Part model, mm, in its own coordinate system. Face numbers are marked on the shaded views. A direction names the side the tool comes from. Round coordinates to 2 decimals unless told otherwise and drop trailing zeros. Order: outer loops, then holes, each group sorted by start corner. A loop starts at its lowest first (then second) coordinate and runs counter-clockwise, first axis right, second up. Notation, with made-up numbers: (-24.5, 65.5) - (-8.5, 65.5) arc R35 cw to (-8.5, 100.5) - close; hole circle Ø3 at (-28.5, 24). An arc over 180 degrees is marked (long way). Return JSON: item names as keys, results as strings. Group by question number.
Item 1: Saw through at A-A on z = 0. List the corners of the cut face in (x, y).
Item 2: Saw through at B-B on x = 0. List the corners of the cut face in (y, z).
Item 3: Tool access for the marked faces 4 and 5: list every direction of +Z, -Z, +X, -X, +Y, -Y with a clear straight run to the whole face (end or side of a thin tool).
Item 4: Probe probe 1 along X at (y, z) = (2.3, -5.75); probe 2 along X at (y, z) = (1.8, -6). List the from-to ranges inside material, lowest first.
Item 5: Drop flat-ended pins along their axis: pin 1 (1.8 mm diameter, centred on x = 4.95, z = 4.95, fed in from +Y); pin 2 (4 mm diameter, centred on x = -4.95, z = -4.95, fed in from -Y); pin 3 (5 mm diameter, centred on x = 0, z = 0, fed in from -Y); pin 4 (1.5 mm diameter, centred on y = 0, z = 4, fed in from -X). Give the stop position or say it passes through.
Item 6: Saw through at C-C on z = -4.25. List the corners of the cut face in (x, y), and give its area (3 significant figures).
Item 7: Saw through at D-D on y = -1.1. List the corners of the cut face in (x, z).
Item 8: Two-plate mould, pull along X, no slides. Class the marked faces 1, 2 and 3: released by +X, released by -X, zero draft, split by the parting line, or undercut.
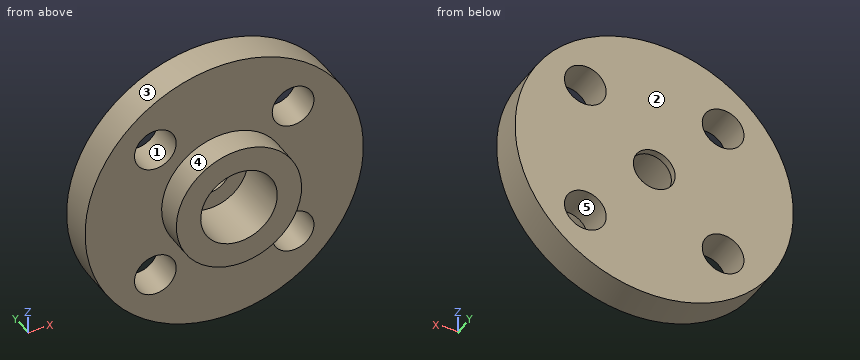
```python
from build123d import *

# Parameters (mm, degrees)
SKETCH_1_R          = 10
SKETCH_1_R_2        = 1.5
EXTRUDE_1_DEPTH     = 2.5
SKETCH_2_R          = 4.5
EXTRUDE_2_DEPTH     = 2
SKETCH_3_R          = 2.75
CUT_EXTRUDE_1_DEPTH = 4


with BuildPart() as part:
    # 草图1 → 凸台-拉伸1 (new body)
    with BuildSketch(Plane(origin=(0, 0, 0), x_dir=(1, 0, 0), z_dir=(0, 1, 0))):
        with Locations(Location((0, 0, 0), (0, 0, 270))):
            Circle(SKETCH_1_R)
        with Locations(Location((0, 0, 0), (0, 0, 270))):
            Circle(SKETCH_1_R_2, mode=Mode.SUBTRACT)
        with Locations(Location((-4.949747468, 4.949747468, 0), (0, 0, 270))):
            Circle(SKETCH_1_R_2, mode=Mode.SUBTRACT)
        with Locations(Location((4.949747468, 4.949747468, 0), (0, 0, 270))):
            Circle(SKETCH_1_R_2, mode=Mode.SUBTRACT)
        with Locations(Location((4.949747468, -4.949747468, 0), (0, 0, 270))):
            Circle(SKETCH_1_R_2, mode=Mode.SUBTRACT)
        with Locations(Location((-4.949747468, -4.949747468, 0), (0, 0, 270))):
            Circle(SKETCH_1_R_2, mode=Mode.SUBTRACT)
    extrude(amount=EXTRUDE_1_DEPTH)

    # 草图2 → 凸台-拉伸2 (add)
    with BuildSketch(Plane.XZ):
        with Locations(Location((0, 0, 0), (0, 0, 90))):
            Circle(SKETCH_2_R)
    extrude(amount=EXTRUDE_2_DEPTH)

    # 草图3 → 切除-拉伸1 (cut)
    with BuildSketch(Plane.XZ.offset(2)):
        with Locations(Location((0, 0, 0), (0, 0, 270))):
            Circle(SKETCH_3_R)
    extrude(amount=-CUT_EXTRUDE_1_DEPTH, mode=Mode.SUBTRACT)


solid = part.part
```
Filled in:
{
 "1": {"outline": "(-10, 0) - (-4.5, 0) - (-4.5, -2) - (-2.75, -2) - (-2.75, 2) - (-1.5, 2) - (-1.5, 2.5) - (-10, 2.5) - close; (1.5, 2) - (2.75, 2) - (2.75, -2) - (4.5, -2) - (4.5, 0) - (10, 0) - (10, 2.5) - (1.5, 2.5) - close"},
 "2": {"outline": "(-2, -4.5) - (0, -4.5) - (0, -10) - (2.5, -10) - (2.5, -1.5) - (2, -1.5) - (2, -2.75) - (-2, -2.75) - close; (-2, 2.75) - (2, 2.75) - (2, 1.5) - (2.5, 1.5) - (2.5, 10) - (0, 10) - (0, 4.5) - (-2, 4.5) - close"},
 "3": {"face 4": "-Y", "face 5": "+Y, -Y"},
 "4": {"probe 1": "x = -8.18 to -6.22, -3.68 to 3.68, 6.22 to 8.18", "probe 2": "x = -8 to -6.02, -3.88 to 3.88, 6.02 to 8"},
 "5": {"pin 1": "passes through", "pin 2": "stops at y = 0", "pin 3": "stops at y = 2", "pin 4": "stops at x = -9.46"},
 "6": {"outline": "(-9.05, 0) - (-6.28, 0) - (-6.28, 2.5) - (-9.05, 2.5) - close; (-3.62, 0) - (-1.48, 0) - (-1.48, -2) - (1.48, -2) - (1.48, 0) - (3.62, 0) - (3.62, 2.5) - (-3.62, 2.5) - close; (6.28, 0) - (9.05, 0) - (9.05, 2.5) - (6.28, 2.5) - close", "area": "37.9 mm^2"},
 "7": {"outline": "circle Ø9 at (0, 0); hole circle Ø5.5 at (0, 0)"},
 "8": {"face 1": "undercut", "face 2": "zero draft", "face 3": "split by the parting line"}
}
